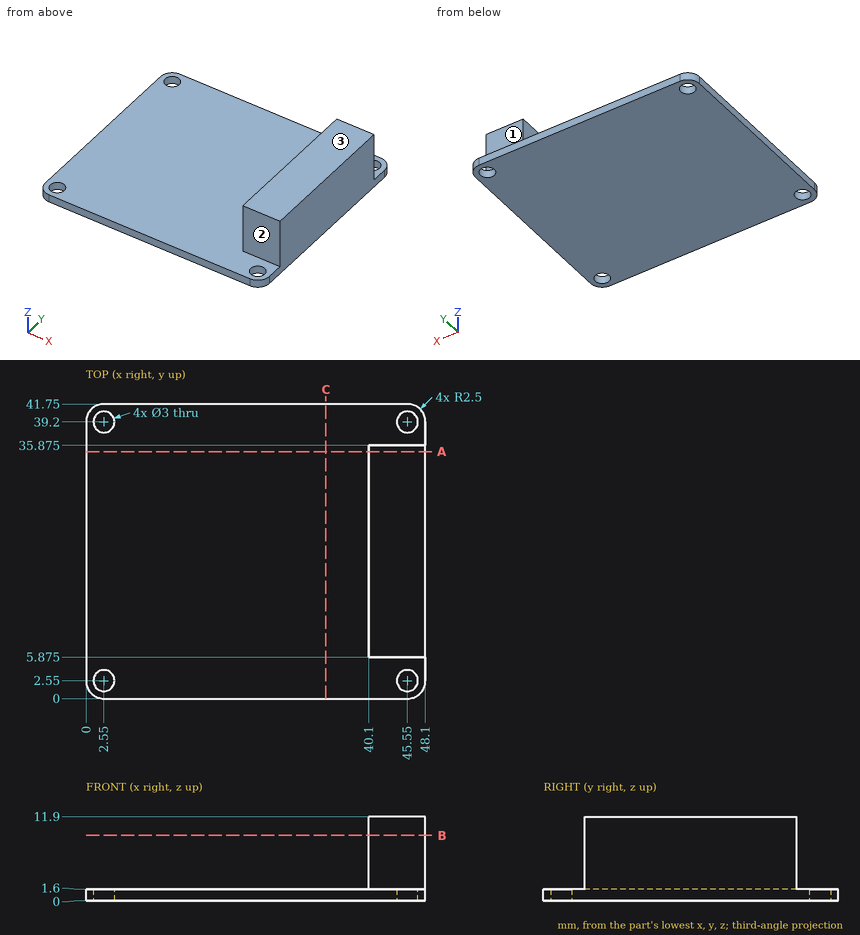
The drawing under review shows one solid part. Ordinate dimensions are in mm from its lowest x, y, z. A direction names the side the tool comes from. Coordinates: 2 decimals unless noted, no trailing zeros. Write each loop counter-clockwise with the first axis right and the second up, starting at its lowest first coordinate (ties: lowest second). Pieces come first, ordered by that corner, then holes. Notation, with made-up numbers: M 48,-11 L 76,-11 A33 cw 76,22 Z; hole C 51,19.25 d8. An arc over 180 degrees is marked long. Put each result on its own line as item: value.
1) Clearance check with flat-ended pins moving along their axes: pin 1 Ø6.5 at (x, z) = (43, 7.5) entering from -Y (3 decimals); pin 2 Ø3.5 at (x, y) = (2.55, 39.2) entering from +Z; pin 3 Ø2.5 at (x, y) = (45.55, 2.55) entering from -Z; pin 4 Ø4 at (x, z) = (45, 8.5) entering from +Y (3 decimals). State where each tip first meets the part, or that it passes through.
Computed:
pin 1: stops at y = 5.875
pin 2: stops at z = 1.6
pin 3: passes through
pin 4: stops at y = 35.875
2) Add section C-C on x = 34. Give the boundary of the cut face in (y, z).
Computed:
outline: M 0,0 L 41.75,0 L 41.75,1.6 L 0,1.6 Z
3) Add section B-B on z = 9.25. Give the boundary of the cut face in (x, y) (3 decimals).
Computed:
outline: M 40.1,5.875 L 48.1,5.875 L 48.1,35.875 L 40.1,35.875 Z
4) For the marked faces 1, 2 and 3, list the 3-axis set-ups (+Z, -Z, +X, -X, +Y, -Y) from which the entire face can be reached by the end or side of a thin tool; tool diameter is ignored.
Computed:
face 1: +Z, +X, -X, +Y
face 2: +Z, +X, -X, -Y
face 3: +Z, +X, -X, +Y, -Y
5) Add section A-A on y = 35. Give the boundary of the cut face in (x, z).
Computed:
outline: M 0,0 L 48.1,0 L 48.1,11.9 L 40.1,11.9 L 40.1,1.6 L 0,1.6 Z
6) Wall thickness on probe 1 along Y at (x, z) = (45, 1.5); probe 2 along X at (y, z) = (2, 1.5); probe 3 along X at (y, z) = (8, 8.5): over which ranges is each line inside the solid? List them lowest first. Write a range as [from, to].
Computed:
probe 1: y = [0, 1.15], [3.95, 37.8], [40.6, 41.75]
probe 2: x = [0.05, 1.15], [3.95, 44.15], [46.95, 48.05]
probe 3: x = [40.1, 48.1]
